Autodesk Inventor part; units mm, degrees
ref_plane "YZ Plane" through (0, 0, 0) normal (1, 0, 0) x (0, 1, 0)
ref_plane "XZ Plane" through (0, 0, 0) normal (0, 1, 0) x (-1, 0, 0)
ref_plane "XY Plane" through (0, 0, 0) normal (0, 0, 1) x (1, 0, 0)
sketch "Sketch1" plane through (0, 0, 0) normal (0, 0, 1) x (1, 0, 0)
  circle A0 centre (0, 0) radius 7.5
  line L0 (-17.5, 0) -> (-7.5, 0)
  line L1 (7.5, 0) -> (17.5, 0)
  line L2 (-17.5, 0) -> (-17.5, 12.5)
  line L3 (-17.5, 12.5) -> (17.5, 12.5)
  line L4 (17.5, 12.5) -> (17.5, 0)
  dimension "d5" = 15
  dimension "d6" = 0
  dimension "d8" = 0
  dimension "d11" = 10
  dimension "d13" = 10
  dimension "d19" = 12.5
  dimension "d76" = 35
extrude "Extrusion1" add sketch "Sketch1" along normal blind 48 contours A0 L0 L2 L3 L4 L1
sketch "Sketch3" plane through (7.5, 0, 0) normal (0, -1, 0) x (1, 0, 0)
  line L0 (10, 0) -> (10, 48)
  line L1 (0, 48) -> (10, 48)
  line L2 (0, 0) -> (0, 48)
  line L3 (0, 0) -> (10, 0)
  line L4 (-25, 0) -> (-15, 0)
  line L5 (-15, 0) -> (-15, 48)
  line L6 (-25, 48) -> (-15, 48)
  line L7 (-25, 0) -> (-25, 48)
  point P0 (-7.5, 0)
  point P1 (5, 4.5)
  point P2 (5, 24)
  point P3 (5, 43.5)
  point P4 (-20, 43.5)
  point P5 (-20, 4.5)
  point P6 (-20, 24)
  dimension "d31" = 48
  dimension "d35" = 5
  dimension "d44" = 4.5
  dimension "d45" = 4.5
  dimension "d46" = 24
  dimension "d47" = 5
  dimension "d48" = 10
  dimension "d49" = 10
hole "Hole1" at (12.5, 0, 4.5) at (12.5, 0, 24) at (12.5, 0, 43.5) at (-12.5, 0, 43.5) at (-12.5, 0, 4.5) at (-12.5, 0, 24) direction (0, 1, 0) diameter 3 end through all
sketch "Sketch4" plane through (17.5, 0, 0) normal (1, 0, 0) x (0, 0, -1)
  line L0 (0, 0) -> (0, 12.5)
  line L1 (0, 12.5) -> (-48, 12.5)
  line L2 (-48, 0) -> (-48, 12.5)
  line L3 (0, 0) -> (-48, 0)
  line L4 (0, 12.5) -> (-48, 12.5)
  circle A0 centre (-33.75, 12.6) radius 3
  circle A1 centre (-14.25, 12.6) radius 3
  dimension "d54" = 6
  dimension "d55" = 6
  dimension "d56" = 14.25
  dimension "d57" = 14.25
  dimension "d58" = 0.1
  dimension "d59" = 0.1
extrude "Extrusion3" cut sketch "Sketch4" against normal through all contours A1 L1 | L1 A1 | A0 L1 | L1 A0
chamfer "Chamfer1" distance 3 angle 45 4 edges at (17.5, 6.25, 48) (-17.5, 6.25, 48) (17.5, 6.25, 0) (-17.5, 6.25, 0)
fillet "Fillet2" radius 2 8 edges at (17.5, 6.25, 45) (14.5, 6.25, 48) (-14.5, 6.25, 48) (-17.5, 6.25, 45) (-17.5, 6.25, 3) (-14.5, 6.25, 0) (14.5, 6.25, 0) (17.5, 6.25, 3)
sketch "Sketch5" plane through (17.5, 12.5, 30.7517) normal (1, 0, 0) x (0, 0, -1)
  line L0 (-17.2483, 0) -> (-17.2483, -12.5)
  line L1 (30.7517, -12.5) -> (30.7517, 0)
  line L2 (26.9232, -12.5) -> (-13.4199, -12.5)
  point P0 (-2.9983, -6.5)
  point P1 (16.5017, -6.5)
  dimension "d66" = 6
  dimension "d67" = 14.25
  dimension "d68" = 14.25
hole "Hole2" at (17.5, 6, 33.75) at (17.5, 6, 14.25) direction (-1, 0, 0) diameter 2.5 depth 10 tip angle 118
equation "\"d13\" = d11"
equation "\"d57\" = d56"
properties part number "3DP_PLA_X_end_top_half" material "ABS Plastic"
Model file for the job. Use its own axes, mm. Give positions to 0.01 mm unless a question says otherwise; leave off trailing zeros. Order: outer loops, then holes, each group sorted by start corner. A loop starts at its lowest first (then second) coordinate and runs counter-clockwise, first axis right, second up. Notation, with made-up numbers: (-2.75, -25.5) - (51.25, -25.5) arc R26 cw to (51.25, -6.5) - close; hole circle Ø3 at (3.5, 38.5). An arc over 180 degrees is marked (long way). Write item = value, one per line. Start each with the question number.
1. Cut at C-C, the plane z = 24. List the corners of the cut face in (x, y).
2. Two-plate mould, pull along X, no slides. Class faces 1 (the cylindrical face through (0.2, 9.6, 33.8)), 2 (the cylindrical face through (13.4, 6.3, 5.7)), 3 (the cylindrical face through (14.447, 6.162, 47.844)): pulls with the +X half, pulls with the -X half, needs draft (parallel to the pull), parting line crosses it, or undercut.
3. Cut at A-A, the plane x = 12.5. List the corners of the cut face in (y, z).
4. Cut at D-D, the plane y = 2.75. List the corners of the cut face in (x, z), and give its area (3 significant figures).
5. Cut at B-B, the plane x = -12.5. List the corners of the cut face in (y, z), and give its area (3 significant figures).
6. Probe line 1 along Z through (x, y) = (-12.5, 3.5); line 2 along Y through (x, z) = (11.25, 33.75); line 3 along Z through (x, y) = (13, 5.5). List the from-to ranges inside material, lowest first.
7. Drop flat-ended pins along their axis: P1, Ø2.5, axis at x = -12.5, z = 24, coming from the +Y side; P2, Ø8, axis at x = -1, z = 5.5, coming from the -Y side; P3, Ø1, axis at x = -11, z = 32, coming from the +Y side. Give the stop position or say it passes through.
Taken from the geometry:
q1.outline = (-17.5, 0) - (-14, 0) - (-14, 12.5) - (-17.5, 12.5) - close; (-11, 0) - (-7.5, 0) arc R7.5 cw to (7.5, 0) - (11, 0) - (11, 12.5) - (-11, 12.5) - close; (14, 0) - (17.5, 0) - (17.5, 12.5) - (14, 12.5) - close
q2.face_1 = needs draft
q2.face_2 = undercut
q2.face_3 = pulls with the +X half
q3.outline = (0, 0) - (12.5, 0) - (12.5, 3) - (0, 3) - close; (0, 6) - (12.5, 6) - (12.5, 11.25) arc R3 cw to (12.5, 17.25) - (12.5, 22.5) - (0, 22.5) - close; (0, 25.5) - (12.5, 25.5) - (12.5, 30.75) arc R3 cw to (12.5, 36.75) - (12.5, 42) - (0, 42) - close; (0, 45) - (12.5, 45) - (12.5, 48) - (0, 48) - close; hole circle Ø2.5 at (6, 14.25); hole circle Ø2.5 at (6, 33.75)
q4.outline = (-17.5, 3.83) arc R2 ccw to (-16.91, 2.41) - (-15.09, 0.59) arc R2 ccw to (-13.67, 0) - (-6.98, 0) - (-6.98, 48) - (-13.67, 48) arc R2 ccw to (-15.09, 47.41) - (-16.91, 45.59) arc R2 ccw to (-17.5, 44.17) - close; (6.98, 0) - (13.67, 0) arc R2 ccw to (15.09, 0.59) - (16.91, 2.41) arc R2 ccw to (17.5, 3.83) - (17.5, 44.17) arc R2 ccw to (16.91, 45.59) - (15.09, 47.41) arc R2 ccw to (13.67, 48) - (6.98, 48) - close; hole circle Ø3 at (-12.5, 4.5); hole circle Ø3 at (-12.5, 24); hole circle Ø3 at (-12.5, 43.5); hole circle Ø3 at (12.5, 4.5); hole circle Ø3 at (12.5, 24); hole circle Ø3 at (12.5, 43.5)
q4.area = 949 mm²
q5.outline = (0, 0) - (12.5, 0) - (12.5, 3) - (0, 3) - close; (0, 6) - (12.5, 6) - (12.5, 11.25) arc R3 cw to (12.5, 17.25) - (12.5, 22.5) - (0, 22.5) - close; (0, 25.5) - (12.5, 25.5) - (12.5, 30.75) arc R3 cw to (12.5, 36.75) - (12.5, 42) - (0, 42) - close; (0, 45) - (12.5, 45) - (12.5, 48) - (0, 48) - close
q5.area = 460 mm²
q6.line_1 = 0 to 3, 6 to 22.5, 25.5 to 42, 45 to 48
q6.line_2 = 0 to 4.75, 7.25 to 9.6
q6.line_3 = 0 to 3.09, 5.91 to 13.1, 15.4 to 22.59, 25.41 to 32.6, 34.9 to 42.09, 44.91 to 48
q7.P1 = through
q7.P2 = 5.59
q7.P3 = 10.62
